Here's how the part is built. I have some questions about the finished solid (model axes, mm). Round coordinates to 2 decimals unless told otherwise and drop trailing zeros. Loops run counter-clockwise (first coordinate to the right, second up) from the corner with the lowest first, then second, coordinate; pieces in that order, holes last. Notation, with made-up numbers: M 15,85.25 L 41,85.25 A13 cw 41,96.25 Z; hole C -18.75,34.25 d6. An arc over 180 degrees is marked long. Write each question's results on one line, items separated by ' | '. Start each with the question number.
Autodesk Inventor part; units mm, degrees
ref_plane "YZ Plane" through (0, 0, 0) normal (1, 0, 0) x (0, 1, 0)
ref_plane "XZ Plane" through (0, 0, 0) normal (0, 1, 0) x (-1, 0, 0)
ref_plane "XY Plane" through (0, 0, 0) normal (0, 0, 1) x (1, 0, 0)
sketch "Sketch2" plane through (0, 0, 0) normal (0, 0, 1) x (1, 0, 0)
  line L0 (0, 0) -> (-10, 0)
  line L1 (-10, 0) -> (-10, 210)
  line L2 (-10, 210) -> (0, 210)
  line L3 (0, 210) -> (0, 0)
  point P0 (-5, 18)
  dimension "d4" = 10
  dimension "d5" = 210
extrude "Extrusion2" add sketch "Sketch2" along normal blind 2
sketch "Sketch3" plane through (0, 0, 2) normal (0, 0, 1) x (1, 0, 0)
  point P0 (0, 0)
  point P1 (-5, 7)
hole "Hole2" at (-5, 7, 2) direction (0, 0, -1) diameter 5 depth 5
properties part number "Circle_TestFit_V1"
Item 1: I need wall thicknesses on L1, parallel to X at y = 7, z = 1.55; L2, parallel to Y at x = -5, z = 0.95. Which ranges of each line are inside material? Lowest first, please.
Item 2: If we mould it in two halves opening along Y, with no side actions, what happens to faces 1 (the face through (-5, 106, 0)), 2 (the face through (-5.751, 4.615, 0.986))? For each: released by +Y, released by -Y, zero draft, split by the parting line, or undercut.
Item 3: If we section it at A-A on x = -5: Please give me the cut outline in (y, z), and give its area (3 significant figures).
Item 4: If we section it at B-B on y = 7: Please give me the cut outline in (x, z), and give its area (3 significant figures).
Numbers:
1) L1: -10 to -7.5, -2.5 to 0 | L2: 0 to 4.5, 9.5 to 210
2) face 1: zero draft | face 2: undercut
3) outline: M 0,0 L 4.5,0 L 4.5,2 L 0,2 Z; M 9.5,0 L 210,0 L 210,2 L 9.5,2 Z | area: 410 mm²
4) outline: M -10,0 L -7.5,0 L -7.5,2 L -10,2 Z; M -2.5,0 L 0,0 L 0,2 L -2.5,2 Z | area: 10.0 mm²
